```python
from build123d import *

# Parameters (mm, degrees)
F0_W     = 50.8
F0_H     = 19.05
F1_DEPTH = 1111.25
F2_W     = 122.435573
F2_H     = 50.8
F2_W_2   = 93.867282
F2_W_3   = 343.160421
F2_H_2   = 127
F3_DEPTH = 25.4
F4_R     = 4.7625
F5_DEPTH = 25.4


with BuildPart() as f1:
    # F0 (on Top) → F1 (new body)
    with BuildSketch(Plane.XY):
        Rectangle(F0_W, F0_H)
    extrude(amount=F1_DEPTH)

    # F2 (on Front) → F3 (cut)
    with BuildSketch(Plane.XZ):
        with Locations((22.446524, 25.4)):
            Rectangle(F2_W, F2_H)
        with Locations((2.720783, 755.65)):
            Rectangle(F2_W_2, F2_H)
        with Locations((-38.781822, 1047.75)):
            Rectangle(F2_W_3, F2_H_2)
    extrude(amount=F3_DEPTH, mode=Mode.SUBTRACT)

    # F4 (on Front) → F5 (cut)
    with BuildSketch(Plane.XZ):
        with Locations((15.875, 254)):
            Circle(F4_R)
        with Locations((15.875, 482.6)):
            Circle(F4_R)
    extrude(amount=F5_DEPTH, mode=Mode.SUBTRACT)


solid = f1.part
```
Check sheet for the modelled part. Datum: model origin and axes. Units: mm. A direction names the side the tool comes from. Round coordinates to 2 decimals unless told otherwise and drop trailing zeros. Order: outer loops, then holes, each group sorted by start corner. A loop starts at its lowest first (then second) coordinate and runs counter-clockwise, first axis right, second up. Notation, with made-up numbers: (16, 79.25) -> (44, 79.25) arc R12 cw to (44, 92.25) -> close; hole circle Ø4 at (-34, -11.5). An arc over 180 degrees is marked (long way). Use CSV: the item, a comma, the result in double quotes.
(1) Draft check along Z on faces 4 (the face through (0, -9.525, 881)), 5 (the face through (0, 0, 756)). Enter one of: pulls with the +Z half, pulls with the -Z half, needs draft (parallel to the pull), parting line crosses it, or undercut.
Worked out:
face 4,"needs draft"
face 5,"undercut"
(2) Cross-section at A-A (y = -4.75). Count the separate pieces of the cut face and the enclosed holes in it, and give its area (3 significant figures).
Worked out:
separate pieces,"2"
enclosed holes,"2"
area,"44,700 mm²"
(3) Cross-section at C-C (z = 757.5). Record the boundary of the cut face in (x, y) (3 decimals).
Worked out:
outline,"(-25.4, 0) -> (25.4, 0) -> (25.4, 9.525) -> (-25.4, 9.525) -> close"
(4) Tool access check on faces 1 (the face through (0, 0, 26)), 2 (the face through (0, 0, 1049)), 3 (the face through (0, -9.525, 386)). Record the directions out of +Z, -Z, +X, -X, +Y, -Y that give a thin tool (end or side, any length) a straight path to the whole face; none if there is none.
Worked out:
face 1,"-Z, +X, -X, -Y"
face 2,"+Z, +X, -X, -Y"
face 3,"+Z, -Z, +X, -X, -Y"
(5) Material ranges on line 1 along Z through (x, y) = (17, -3.5); line 2 along Z through (x, y) = (10.5, -8.5); line 3 along Z through (x, y) = (13, -5.5), recorded low to high. Write a range as from..to.
Worked out:
line 1,"50.8..249.37, 258.63..477.97, 487.23..730.25, 781.05..984.25"
line 2,"50.8..730.25, 781.05..984.25"
line 3,"50.8..250.2, 257.8..478.8, 486.4..730.25, 781.05..984.25"
(6) Depth check by flat-ended pin: pin 1 (15 mm diameter, centred on x = -7.5, z = 744, fed in from -Y); pin 2 (7.5 mm diameter, centred on x = -1.5, y = -6, fed in from +Z). Enter the tip coordinate at first touch or a pass-through.
Worked out:
pin 1,"y = 0"
pin 2,"z = 984.25"
(7) Cross-section at B-B (x = -9). Record the boundary of the cut face in (y, z) (3 decimals).
Worked out:
outline,"(-9.525, 50.8) -> (0, 50.8) -> (0, 0) -> (9.525, 0) -> (9.525, 1111.25) -> (0, 1111.25) -> (0, 984.25) -> (-9.525, 984.25) -> (-9.525, 781.05) -> (0, 781.05) -> (0, 730.25) -> (-9.525, 730.25) -> close"
